Part print with two shaded views. Sizes in mm from the minimum x, y, z corner. A direction names the side the tool comes from. Coordinates: 2 decimals unless noted, no trailing zeros. Loops run counter-clockwise (first coordinate to the right, second up) from the corner with the lowest first, then second, coordinate; pieces in that order, holes last. Notation, with made-up numbers: (79, 88.25) -> (133, 88.25) arc R26 cw to (133, 116.25) -> close; hole circle Ø10 at (4, 34). An arc over 180 degrees is marked (long way). One line per item, written item: value. Start each with the question number.
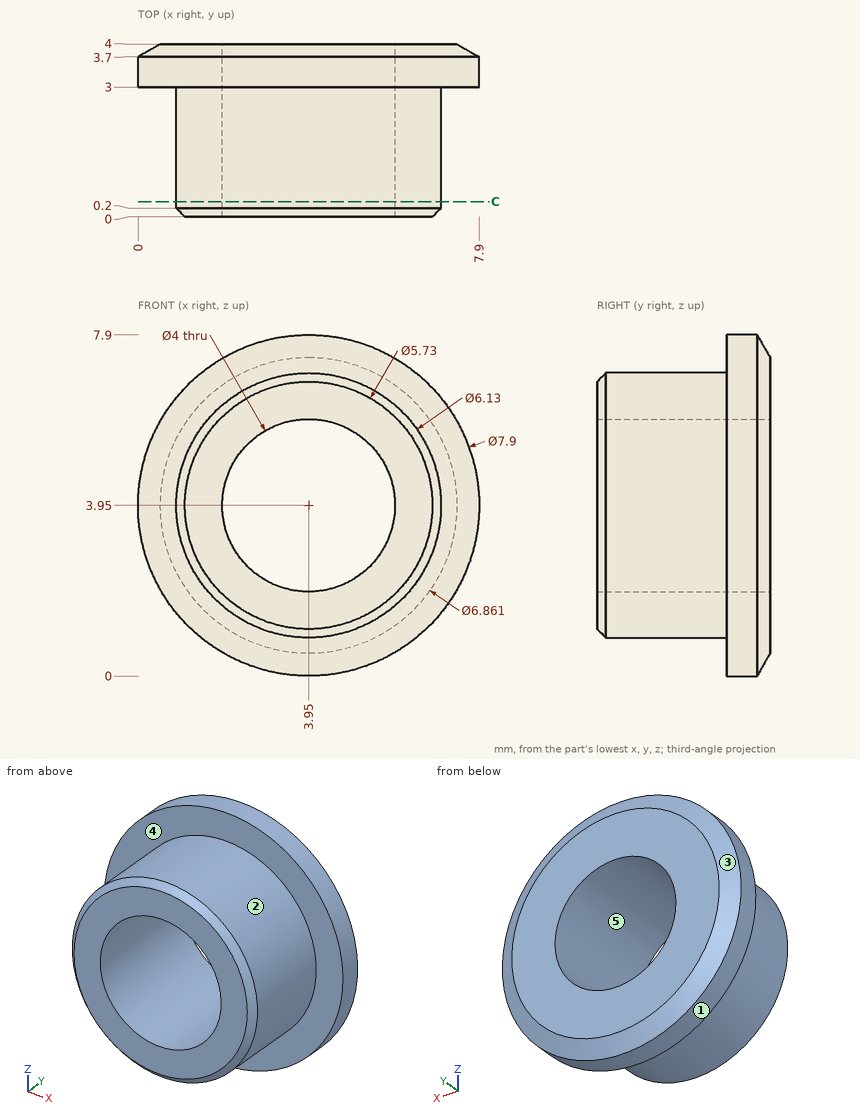
Item 1: Probe probe 1 along X at (y, z) = (2.95, 3.95) (3 decimals); probe 2 along Y at (x, z) = (6.75, 5.5); probe 3 along Z at (x, y) = (2.25, 1.4) (1 decimal). List the from-to ranges inside material, lowest first.
Item 2: Two-plate mould, pull along X, no slides. Class the marked faces 3, 4 and 5: +X half, -X half, draft (parallel to the pull), parting line (faces both ways), or undercut.
Item 3: Band-saw the part on C-C, the plane y = 0.35. List the corners of the cut face in (x, z) (3 decimals).
Item 4: Tool access for the marked faces 1 and 2: list every direction of +Z, -Z, +X, -X, +Y, -Y with a clear straight run to the whole face (end or side of a thin tool).
Item 5: Drop a flat-ended pin along its axis: pin 1 Ø1 at (y, z) = (3.5, 1) entering from +X. Give the stop position or say it passes through.
Worked out:
1. probe 1: x = 0.885 to 1.95, 5.95 to 7.015
1. probe 2: y = 3 to 4
1. probe 3: z = 1.4 to 2.9, 5 to 6.5
2. face 3: parting line
2. face 4: draft
2. face 5: undercut
3. outline: circle Ø6.13 at (3.95, 3.95); hole circle Ø4 at (3.95, 3.95)
4. face 1: +Y, -Y
4. face 2: -Y
5. pin 1: stops at x = 7.05
